Model file for the job. Use its own axes, mm. A direction names the side the tool comes from. Coordinates: 2 decimals unless noted, no trailing zeros. Loops run counter-clockwise (first coordinate to the right, second up) from the corner with the lowest first, then second, coordinate; pieces in that order, holes last.
from build123d import *

# Parameters (mm, degrees)
SKETCH1_W           = 23
SKETCH1_H           = 23
BOSS_EXTRUDE1_DEPTH = 10
CUT_EXTRUDE1_DEPTH  = 24
SKETCH3_R           = 2.2
CUT_EXTRUDE2_DEPTH  = 5.3


with BuildPart() as part:
    # Sketch1 → Boss-Extrude1 (new body)
    with BuildSketch(Plane(origin=(0, 0, 0), x_dir=(1, 0, 0), z_dir=(0, 1, 0))):
        Rectangle(SKETCH1_W, SKETCH1_H)
    extrude(amount=BOSS_EXTRUDE1_DEPTH)

    # Sketch2 → Cut-Extrude1 (cut, through all)
    with BuildSketch(Plane.XY.offset(11.5)):
        with BuildLine():
            Line((-2.5, 0), (-0.15607285, 2.925065045))
            ThreePointArc((-0.15607285, 2.925065045), (0, 3), (0.15607285, 2.925065045))
            Line((0.15607285, 2.925065045), (2.5, 0))
            Line((2.5, 0), (-2.5, 0))
        make_face()
    extrude(amount=-CUT_EXTRUDE1_DEPTH, mode=Mode.SUBTRACT)

    # Sketch3 → Cut-Extrude2 (cut)
    with BuildSketch(Plane.XZ):
        Circle(SKETCH3_R)
    extrude(amount=-CUT_EXTRUDE2_DEPTH, mode=Mode.SUBTRACT)


solid = part.part
Q1. Drill centre lines: line 1 (X direction, y = 4.3, z = 0); line 2 (X direction, y = 0.75, z = -6.5). Where is each one in solid material? Low to high.
Answers:
line 1: x = -11.5 to -2.2, 2.2 to 11.5
line 2: x = -11.5 to -1.9, 1.9 to 11.5
Q2. Slice it at A-A (y = 1.75). List the corners of the cut face in (x, z), and give its area (3 significant figures).
Answers:
outline: (-11.5, -11.5) - (-1.1, -11.5) - (-1.1, -1.91) arc R2.2 cw to (-1.1, 1.91) - (-1.1, 11.5) - (-11.5, 11.5) - close; (1.1, -11.5) - (11.5, -11.5) - (11.5, 11.5) - (1.1, 11.5) - (1.1, 1.91) arc R2.2 cw to (1.1, -1.91) - close
area: 473 mm2
Q3. Slice it at C-C (z = 0). List the corners of the cut face in (x, y).
Answers:
outline: (-11.5, 0) - (-2.5, 0) - (-2.2, 0.37) - (-2.2, 5.3) - (2.2, 5.3) - (2.2, 0.37) - (2.5, 0) - (11.5, 0) - (11.5, 10) - (-11.5, 10) - close
Q4. Which spindle directions (+Z, -Z, +X, -X, +Y, -Y) get a long thin tool onto all of the face, cutting with end or side? Do faces 4 (the cylindrical face through (1.183, 3.35, 1.855)), 5 (the flat face through (-11.5, 5, 0)), 6 (the flat face through (2.353, 0.183, 0.161)). Say none if no direction does.
Answers:
face 4: -Y
face 5: +Z, -Z, -X, +Y, -Y
face 6: +Z, -Z, -Y
Q5. Mould opens along X. For faces 1 (the flat face through (0, 5.3, 0)), 2 (the flat face through (-7, 0, 0)), 3 (the flat face through (11.5, 5, 0)) say: +X half, -X half, draft (parallel to the pull), parting line (faces both ways), or undercut.
Answers:
face 1: undercut
face 2: draft
face 3: +X half
Q6. Flat gauge pins, fed straight in: P1, Ø1, axis at x = 0, z = 6.5, coming from the -Y side; P2, Ø2, axis at x = -0.5, z = 0, coming from the -Y side. Where does each tip first touch, or does it go through?
Answers:
P1: stops at y = 2.5
P2: stops at y = 5.3
Q7. Slice it at B-B (z = 9). List the corners of the cut face in (x, y), and give its area (3 significant figures).
Answers:
outline: (-11.5, 0) - (-2.5, 0) - (-0.16, 2.93) arc R0.2 cw to (0.16, 2.93) - (2.5, 0) - (11.5, 0) - (11.5, 10) - (-11.5, 10) - close
area: 222 mm2
